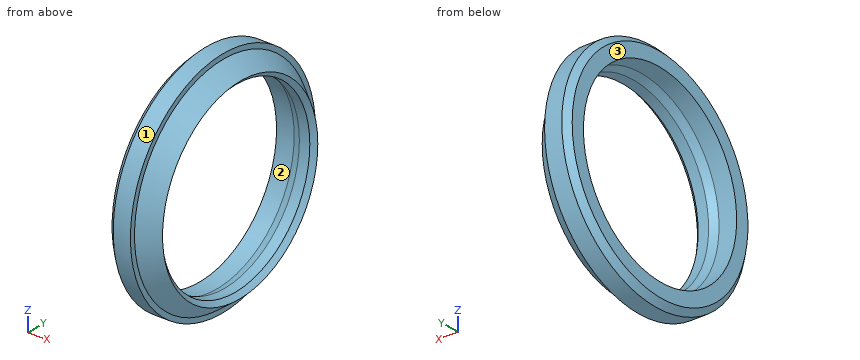
Autodesk Inventor part; units mm, degrees
ref_plane "YZ Plane" through (0, 0, 0) normal (1, 0, 0) x (0, 1, 0)
ref_plane "XZ Plane" through (0, 0, 0) normal (0, 1, 0) x (-1, 0, 0)
ref_plane "XY Plane" through (0, 0, 0) normal (0, 0, 1) x (1, 0, 0)
sketch "Sketch1" plane through (0, 0, 0) normal (0, 0, 1) x (1, 0, 0)
  line L0 (4, 19.1204) -> (4, 20)
  line L1 (4, 20) -> (0, 20)
  line L2 (0, 20) -> (0, 16.5676)
  line L3 (0, 16.5676) -> (3.0669, 16.5676)
  line L4 (3.0669, 16.5676) -> (4.4257, 16)
  line L5 (4.4257, 16) -> (6.2458, 16)
  line L6 (6.2458, 16) -> (7, 16.7884)
  line L7 (7, 16.7884) -> (4, 19.1204)
  line L8 (0, 0) -> (20.4487, 0)
  dimension "d0" = 84.13
  dimension "d1" = 133.729
  dimension "d2" = 111.058
  dimension "d3" = 4
  dimension "d4" = 0.5675
  dimension "d5" = 4
  dimension "d6" = 0.7884
  dimension "d7" = 3
  dimension "d8" = 1.7197
  dimension "d9" = 32
revolve "Revolution1" add sketch "Sketch1" angle 360 about axis through (0, 0, 0) along (1, 0, 0)
chamfer "Fase1" distance 1 angle 45 1 edges at (0, -20, 0)
properties part number "Collar_Seal_Outer" material "Nylon-6/6"
The listing builds one solid part. Answer for the finished solid, in the listing's coordinates (mm). Face numbers are marked on the shaded views. Coordinates: 2 decimals unless noted, no trailing zeros. Write each loop counter-clockwise with the first axis right and the second up, starting at its lowest first coordinate (ties: lowest second). Pieces come first, ordered by that corner, then holes. Notation, with made-up numbers: (55.5, 22.5) - (88.5, 22.5) arc R13 cw to (88.5, 28.5) - close; hole circle Ø9 at (-34, -27.5). An arc over 180 degrees is marked (long way). One line per item, written item: value.
1) Find section A-A (y = 0). Give the vertices of the cut face in (x, z), and give its area (3 significant figures).
Geometry check:
outline: (0, -19) - (1, -20) - (4, -20) - (4, -19.12) - (7, -16.79) - (6.25, -16) - (4.43, -16) - (3.07, -16.57) - (0, -16.57) - close; (0, 16.57) - (3.07, 16.57) - (4.43, 16) - (6.25, 16) - (7, 16.79) - (4, 19.12) - (4, 20) - (1, 20) - (0, 19) - close
area: 37.9 mm2
2) Each of these flat-tipped pins is pushed along its axis until it touches: pin 1 Ø4 at (x, y) = (5.5, -10.5) entering from +Z; pin 2 Ø1 at (y, z) = (-15.5, 13) entering from -X; pin 3 Ø4 at (x, z) = (4.5, -14.5) entering from -Y. Where does it stop, or does it pass through?
Geometry check:
pin 1: stops at z = 17.77
pin 2: stops at x = 0.73
pin 3: stops at y = -15.56
3) Consider line 1 along Z through (x, y) = (1.1, 0); line 2 along Z through (x, y) = (3.75, 7.5); line 3 along Y through (x, z) = (4.25, -11). Determine where each line is inside the solid, lowest interval first. Write a range as from..to.
Geometry check:
line 1: z = -20..-16.57, 16.57..20
line 2: z = -18.54..-14.45, 14.45..18.54
line 3: y = -15.4..-11.72, 11.72..15.4
4) Find section C-C (x = 1.5). Give the vertices of the cut face in (y, z).
Geometry check:
outline: circle Ø40 at (0, 0); hole circle Ø33.14 at (0, 0)
5) For a pull along Z with two mould halves and no side action, classify the marked faces 1, 2 and 3 as pulls with the +Z half, pulls with the -Z half, needs draft (parallel to the pull), parting line crosses it, or undercut.
Geometry check:
face 1: parting line crosses it
face 2: undercut
face 3: needs draft
